from build123d import *

# Parameters (mm, degrees)
SKETCH1_W           = 63.5
SKETCH1_H           = 38.1
BOSS_EXTRUDE1_DEPTH = 25.4
SKETCH3_W           = 44.45
SKETCH3_H           = 30.48
CUT_EXTRUDE1_DEPTH  = 38.1
SKETCH5_R           = 3.175
CUT_EXTRUDE2_DEPTH  = 76.2
FILLET3_R           = 1.27
SKETCH6_W           = 12.7
SKETCH6_H           = 2.54
BOSS_EXTRUDE2_DEPTH = 7.62
SKETCH7_W           = 12.7
SKETCH7_H           = 2.54
BOSS_EXTRUDE3_DEPTH = 7.62
CUT_EXTRUDE3_REACH  = 4.54
SKETCH8_R           = 3.175
CUT_EXTRUDE4_REACH  = 4.54
SKETCH9_R           = 3.175
FILLET4_R           = 1.27


with BuildPart() as part:
    # Sketch1 → Boss-Extrude1 (new body)
    with BuildSketch(Plane.XY):
        with Locations((31.75, 19.05)):
            Rectangle(SKETCH1_W, SKETCH1_H)
    extrude(amount=BOSS_EXTRUDE1_DEPTH)

    # Sketch3 → Cut-Extrude1 (cut)
    with BuildSketch(Plane(origin=(0, 0, 0), x_dir=(-1, 0, 0), z_dir=(0, 0, -1))):
        with Locations((-41.275, 19.05)):
            Rectangle(SKETCH3_W, SKETCH3_H)
    extrude(amount=-CUT_EXTRUDE1_DEPTH, mode=Mode.SUBTRACT)

    # Sketch5 → Cut-Extrude2 (cut)
    with BuildSketch(Plane.XZ):
        with Locations((44.45, 12.7)):
            Circle(SKETCH5_R)
    extrude(amount=-CUT_EXTRUDE2_DEPTH, mode=Mode.SUBTRACT)

    # Fillet3
    fillet3_edges = [part.edges().sort_by_distance(p)[0] for p in [
        (63.5, 3.81, 12.7),
        (63.5, 34.29, 12.7),
        (19.05, 34.29, 12.7),
        (19.05, 3.81, 12.7),
        (0, 38.1, 12.7),
        (63.5, 38.1, 12.7),
        (63.5, 0, 12.7),
        (0, 0, 12.7),
    ]]
    fillet(fillet3_edges, radius=FILLET3_R)

    # Sketch6 → Boss-Extrude2 (add)
    with BuildSketch(Plane(origin=(0, 38.1, 0), x_dir=(1, 0, 0), z_dir=(0, 1, 0))):
        with Locations((31.75, -24.13)):
            Rectangle(SKETCH6_W, SKETCH6_H)
    extrude(amount=BOSS_EXTRUDE2_DEPTH)

    # Sketch7 → Boss-Extrude3 (add)
    with BuildSketch(Plane.XZ):
        with Locations((31.75, 24.13)):
            Rectangle(SKETCH7_W, SKETCH7_H)
    extrude(amount=BOSS_EXTRUDE3_DEPTH)

    # Sketch8 → Cut-Extrude3 (cut, up to next)
    with BuildSketch(Plane(origin=(0, 0, 22.86), x_dir=(-1, 0, 0), z_dir=(0, 0, -1)), mode=Mode.PRIVATE) as cut_extrude3_sk1:
        with Locations((-31.75, -3.81)):
            Circle(SKETCH8_R)
    cut_extrude3_tool1 = extrude(cut_extrude3_sk1.sketch, amount=-CUT_EXTRUDE3_REACH, mode=Mode.PRIVATE) & part.part
    add(cut_extrude3_tool1.solids().sort_by_distance((31.75, -3.81, 22.86))[0], mode=Mode.SUBTRACT)

    # Sketch9 → Cut-Extrude4 (cut, up to next)
    with BuildSketch(Plane(origin=(0, 0, 22.86), x_dir=(-1, 0, 0), z_dir=(0, 0, -1)), mode=Mode.PRIVATE) as cut_extrude4_sk1:
        with Locations((-31.75, 41.91)):
            Circle(SKETCH9_R)
    cut_extrude4_tool1 = extrude(cut_extrude4_sk1.sketch, amount=-CUT_EXTRUDE4_REACH, mode=Mode.PRIVATE) & part.part
    add(cut_extrude4_tool1.solids().sort_by_distance((31.75, 41.91, 22.86))[0], mode=Mode.SUBTRACT)

    # Fillet4
    fillet4_edges = [part.edges().sort_by_distance(p)[0] for p in [
        (25.4, -7.62, 24.13),
        (38.1, -7.62, 24.13),
        (25.4, 45.72, 24.13),
        (38.1, 45.72, 24.13),
    ]]
    fillet(fillet4_edges, radius=FILLET4_R)


solid = part.part
Can you work these out from the model? Positions are in its coordinate system, mm. A direction names the side the tool comes from. Give positions to 0.01 mm unless a question says otherwise; leave off trailing zeros. Order: outer loops, then holes, each group sorted by start corner. A loop starts at its lowest first (then second) coordinate and runs counter-clockwise, first axis right, second up. Notation, with made-up numbers: M -12.75,21 L -5.75,21 A20 ccw -5.75,55 Z; hole C 54,63 d8. An arc over 180 degrees is marked long. Use a Markdown table: item, result. Add a question column.
Item 1: For faces 1 (the flat face through (38.1, 41, 24)), 2 (the flat face through (25.4, 41, 24)), 3 (the flat face through (29, 40, 22.86)), 4 (the flat face through (19.05, 19, 13)), which set-ups out of +Z, -Z, +X, -X, +Y, -Y let a thin tool reach every point of the face, with its end or its side?
Item 2: If I drill on L1, parallel to Y at x = 33.5, z = 22; L2, parallel to Y at x = 31.75, z = 24 (3 decimals); L3, parallel to Z at x = 44.45, y = 36.9 (3 decimals), over which ranges is the centre line in solid material (lowest first)? Write a range as [from, to].
Item 3: Suppose I cut it at A-A (y = 41.91). List the corners of the cut face in (x, z) for me (3 decimals).
Item 4: We'd pull the mould along Z, two halves only. Please class faces 5 (the flat face through (17, 19, 25.4)), 6 (the cylindrical face through (41.28, 36.17, 12.84)), 7 (the flat face through (17, 19, 0)), 8 (the flat face through (0, 19, 13)): +Z half, -Z half, draft (parallel to the pull), parting line (faces both ways), or undercut.
Item 5: Suppose I cut it at C-C (x = 59.5). List the corners of the cut face in (y, z) for me, then the cut area to 3 significant figures.
Item 6: Suppose I cut it at B-B (x = 44.45). List the corners of the cut face in (y, z) for me (3 decimals).
Item 7: Suppose I cut it at D-D (z = 11.5). List the corners of the cut face in (x, y) for me.
Item 8: Will these pins go through, and if not, where does the flat tip stop? pin 1 (1.5 mm diameter, centred on x = 34.5, z = 16.5, fed in from +Y); pin 2 (8 mm diameter, centred on y = 23, z = 18, fed in from +X); pin 3 (12.5 mm diameter, centred on x = 37.5, z = 7.5, fed in from -Y).
Answer sheet:
| question | item | result |
|---|---|---|
| 1 | face 1 | +Z, -Z, +X, +Y |
| 1 | face 2 | +Z, -Z, -X, +Y |
| 1 | face 3 | -Z, +X, -X, +Y |
| 1 | face 4 | +Z, -Z, +X |
| 2 | L1 | y = [0, 3.81], [34.29, 38.1] |
| 2 | L2 | y = [-7.62, -6.985], [-0.635, 3.81], [34.29, 38.735], [45.085, 45.72] |
| 2 | L3 | z = [0, 9.525], [15.875, 25.4] |
| 3 | outline | M 25.4,22.86 L 28.575,22.86 L 28.575,25.4 L 25.4,25.4 Z; M 34.925,22.86 L 38.1,22.86 L 38.1,25.4 L 34.925,25.4 Z |
| 4 | face 5 | +Z half |
| 4 | face 6 | undercut |
| 4 | face 7 | -Z half |
| 4 | face 8 | draft |
| 5 | outline | M 0,0 L 3.81,0 L 3.81,25.4 L 0,25.4 Z; M 34.29,0 L 38.1,0 L 38.1,25.4 L 34.29,25.4 Z |
| 5 | area | 194 mm² |
| 6 | outline | M 0,0 L 3.81,0 L 3.81,9.525 L 0,9.525 Z; M 0,15.875 L 3.81,15.875 L 3.81,25.4 L 0,25.4 Z; M 34.29,0 L 38.1,0 L 38.1,9.525 L 34.29,9.525 Z; M 34.29,15.875 L 38.1,15.875 L 38.1,25.4 L 34.29,25.4 Z |
| 7 | outline | M 0,1.27 A1.27 ccw 1.27,0 L 41.51,0 L 41.51,3.81 L 20.32,3.81 A1.27 cw 19.05,5.08 L 19.05,33.02 A1.27 cw 20.32,34.29 L 41.51,34.29 L 41.51,38.1 L 1.27,38.1 A1.27 ccw 0,36.83 Z; M 47.39,0 L 62.23,0 A1.27 ccw 63.5,1.27 L 63.5,2.54 A1.27 ccw 62.23,3.81 L 47.39,3.81 Z; M 47.39,34.29 L 62.23,34.29 A1.27 ccw 63.5,35.56 L 63.5,36.83 A1.27 ccw 62.23,38.1 L 47.39,38.1 Z |
| 8 | pin 1 | stops at y = 38.1 |
| 8 | pin 2 | stops at x = 19.05 |
| 8 | pin 3 | stops at y = 0 |
